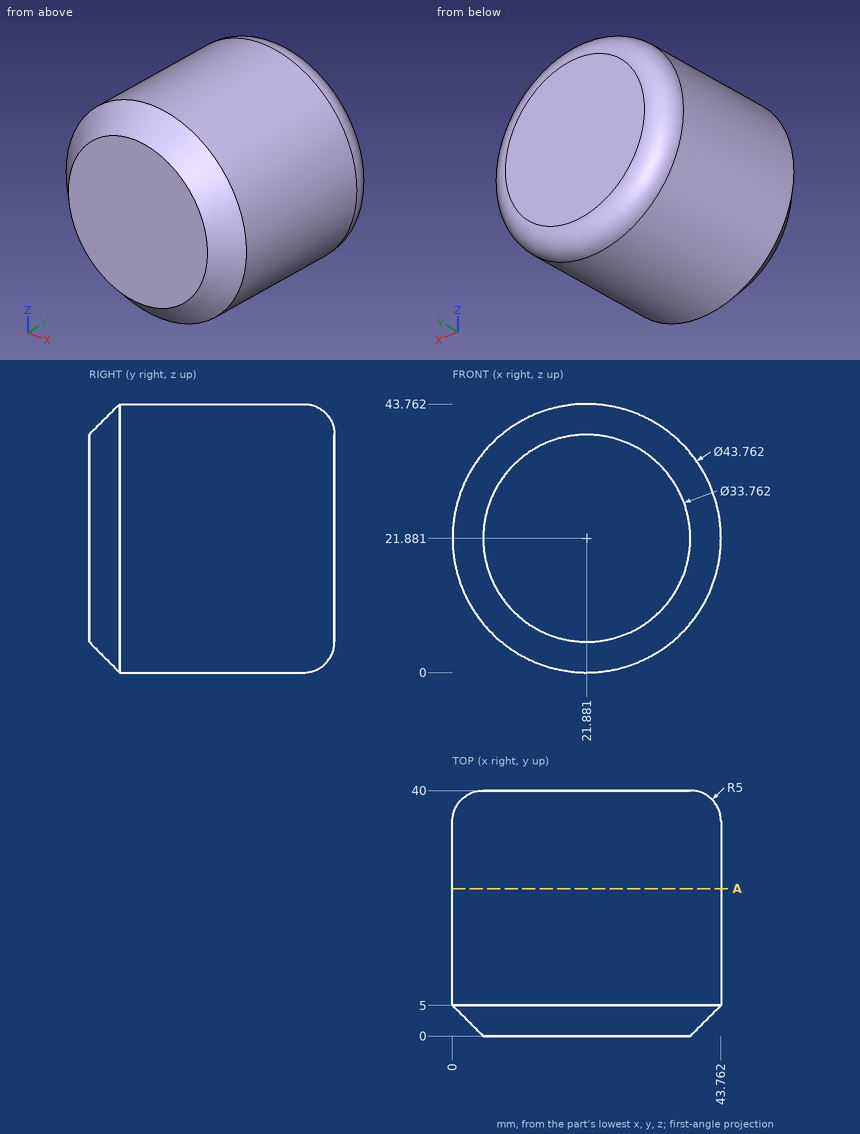
For this review, use the dimensioned drawing (mm, ordinates from the lowest corner) and the shaded views. Round coordinates to 2 decimals unless told otherwise and drop trailing zeros. Write each loop counter-clockwise with the first axis right and the second up, starting at its lowest first coordinate (ties: lowest second). Pieces come first, ordered by that corner, then holes. Notation, with made-up numbers: (36.25, -21) -> (66.25, -21) arc R7 ccw to (66.25, -15) -> close; hole circle Ø10 at (50.25, 50.25). An arc over 180 degrees is marked (long way). One line per item, written item: value. Start each with the question number.
Q1. Insertion check: P1, Ø8, axis at y = 16.5, z = 19.5, coming from the -X side; P2, Ø5, axis at x = 6.5, z = 7.5, coming from the -Y side (1 decimal); P3, Ø1.5, axis at y = 14, z = 4.5, coming from the -X side; P4, Ø3, axis at x = 33, y = 9.5, coming from the -Z side. Each pin has a flat end and moves straight along its axis. Give the tip position at first contact, or say it passes through.
Q2. To check wall thickness, follow probe 1 along X at (y, z) = (26.5, 22); probe 2 along X at (y, z) = (5, 30); probe 3 along Z at (x, y) = (19, 11.5). State the ranges of each line that lie inside material, in increasing order.
Q3. Add section A-A (y = 24). Give the boundary of the cut face in (x, z), then the cut area to 3 significant figures.
Response:
1. P1: stops at x = 0
1. P2: stops at y = 1.7
1. P3: stops at x = 7.66
1. P4: stops at z = 2.23
2. probe 1: x = 0 to 43.76
2. probe 2: x = 1.56 to 42.2
2. probe 3: z = 0.19 to 43.57
3. outline: circle Ø43.76 at (21.88, 21.88)
3. area: 1,500 mm^2
